Check sheet for the drawn part. Datum: minimum x, y, z corner. Units: mm. Coordinates: 2 decimals unless noted, no trailing zeros. Write each loop counter-clockwise with the first axis right and the second up, starting at its lowest first coordinate (ties: lowest second). Pieces come first, ordered by that corner, then holes. Notation, with made-up numbers: (46.5, -17) - (94.5, -17) arc R23 ccw to (94.5, 2) - close; hole circle Ø2 at (62.25, -9). An arc over 180 degrees is marked (long way). Write each question's results on one line, items separated by ' | '.
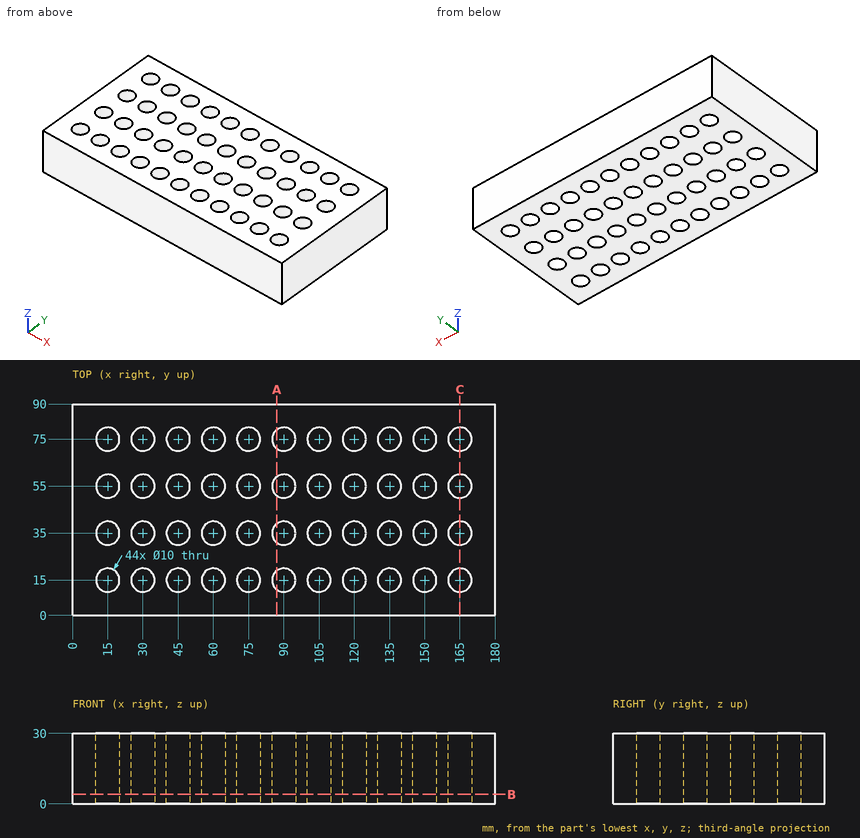
1. Sectioned sample at A-A (x = 87). Record the cut outline in (y, z), then the cut area to 3 significant figures.
Values follow:
outline: (0, 0) - (11, 0) - (11, 30) - (0, 30) - close; (19, 0) - (31, 0) - (31, 30) - (19, 30) - close; (39, 0) - (51, 0) - (51, 30) - (39, 30) - close; (59, 0) - (71, 0) - (71, 30) - (59, 30) - close; (79, 0) - (90, 0) - (90, 30) - (79, 30) - close | area: 1,740 mm^2
2. Go/stop test with a flat-tipped pin: pin 1 (9 mm diameter, centred on x = 60, y = 15, fed in from +Z). Record where the tip stops, or that it passes through.
Values follow:
pin 1: passes through
3. Material ranges on L1, parallel to Y at x = 30, z = 15.75; L2, parallel to Y at x = 133, z = 17.75, recorded low to high. Write a range as [from, to].
Values follow:
L1: y = [0, 10], [20, 30], [40, 50], [60, 70], [80, 90] | L2: y = [0, 10.42], [19.58, 30.42], [39.58, 50.42], [59.58, 70.42], [79.58, 90]
4. Sectioned sample at C-C (x = 165). Record the cut outline in (y, z), then the cut area to 3 significant figures.
Values follow:
outline: (0, 0) - (10, 0) - (10, 30) - (0, 30) - close; (20, 0) - (30, 0) - (30, 30) - (20, 30) - close; (40, 0) - (50, 0) - (50, 30) - (40, 30) - close; (60, 0) - (70, 0) - (70, 30) - (60, 30) - close; (80, 0) - (90, 0) - (90, 30) - (80, 30) - close | area: 1,500 mm^2
5. Sectioned sample at B-B (z = 4). Give the number of separate pieces and of enclosed holes in the cut face, then the cut area to 3 significant figures.
Values follow:
separate pieces: 1 | enclosed holes: 44 | area: 12,700 mm^2
